Part model, mm, in its own coordinate system. Face numbers are marked on the shaded views. A direction names the side the tool comes from. Give positions to 0.01 mm unless a question says otherwise; leave off trailing zeros. Order: outer loops, then holes, each group sorted by start corner. A loop starts at its lowest first (then second) coordinate and runs counter-clockwise, first axis right, second up. Notation, with made-up numbers: (-40, 62.25) - (-14, 62.25) arc R18 ccw to (-14, 88.25) - close; hole circle Ø3 at (80, 66). An arc over 180 degrees is marked (long way). One line per item, written item: value.
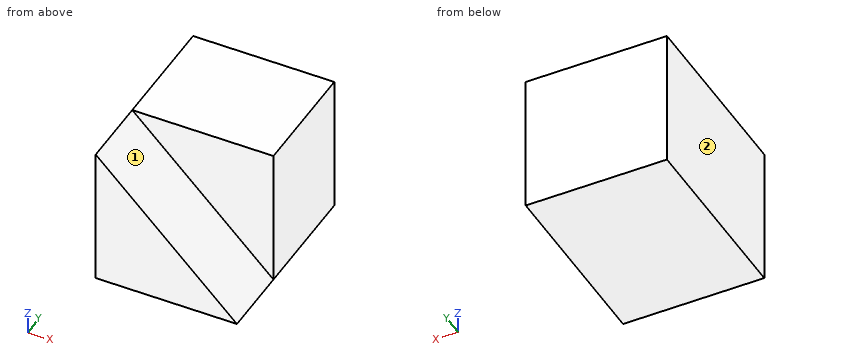
```python
from build123d import *

# Parameters (mm, degrees)
F1_DEPTH = 15
F3_W     = 30
F3_H     = 30
F4_DEPTH = 25


with BuildPart() as f1:
    # F0 (on Front) → F1 (new body)
    with BuildSketch(Plane.XZ):
        Polygon((0, 30), (0, 0), (30, 0), align=None)
    extrude(amount=-F1_DEPTH)

    # F3 (on offset) → F4 (join)
    with BuildSketch(Plane.XZ.offset(-15)):
        with Locations((15, 15)):
            Rectangle(F3_W, F3_H)
    extrude(amount=-F4_DEPTH)


solid = f1.part
```
1) Which spindle directions (+Z, -Z, +X, -X, +Y, -Y) get a long thin tool onto all of the face, cutting with end or side? Do the marked faces 1 and 2. Say none if no direction does.
Answer:
face 1: +Z, +X, -Y
face 2: +Z, -Z, -X, +Y, -Y
2) Slice it at B-B on x = 6. Write the cut outline in (y, z), then the cut area to 3 significant figures.
Answer:
outline: (0, 0) - (40, 0) - (40, 30) - (15, 30) - (15, 24) - (0, 24) - close
area: 1,110 mm2
3) Drop flat-ended pins along their axis: P1, Ø1.5, axis at y = 10, z = 8, coming from the +X side; P2, Ø6, axis at x = 23.5, z = 23, coming from the -Y side. Give the stop position or say it passes through.
Answer:
P1: stops at x = 22.75
P2: stops at y = 15
4) Slice it at C-C on y = 13.5. Write the cut outline in (x, z), then the cut area to 3 significant figures.
Answer:
outline: (0, 0) - (30, 0) - (0, 30) - close
area: 450 mm2
5) Slice it at A-A on z = 20.5. Write the cut outline in (x, y).
Answer:
outline: (0, 0) - (9.5, 0) - (9.5, 15) - (30, 15) - (30, 40) - (0, 40) - close
6) Wall check: line 1 along Y through (x, z) = (24, 28.5); line 2 along Z through (x, y) = (12, 12); line 3 along Z through (x, y) = (4, 2.5). Give the ranges that are in metal, low to high. Write a range as [from, to].
Answer:
line 1: y = [15, 40]
line 2: z = [0, 18]
line 3: z = [0, 26]
